from build123d import *

# Parameters (mm, degrees)
PAD_DEPTH    = 2
SKETCH001_R  = 4.2
POCKET_DEPTH = 1.1


with BuildPart() as part:
    # Sketch → Pad (new body)
    with BuildSketch(Plane.XY):
        with BuildLine():
            ThreePointArc((-47.293619, 36.923077), (0, -60), (47.293619, 36.923077))
            ThreePointArc((47.293619, 123.076923), (32.469508, 80), (47.293619, 36.923077))
            ThreePointArc((47.293619, 123.076923), (0, 220), (-47.293619, 123.076923))
            ThreePointArc((-47.293619, 36.923077), (-32.469508, 80), (-47.293619, 123.076923))
        make_face()
    extrude(amount=PAD_DEPTH)

    # Sketch001 (on Face6 of Pad) → Pocket (cut)
    with BuildSketch(Plane.XY.offset(2)):
        with Locations((0, -54.5)):
            Circle(SKETCH001_R)
        with Locations((0, 214.5)):
            Circle(SKETCH001_R)
        with Locations((0, 80)):
            Circle(SKETCH001_R)
    extrude(amount=-POCKET_DEPTH, mode=Mode.SUBTRACT)


solid = part.part
The listing builds one solid part. Answer for the finished solid, in the listing's coordinates (mm). A direction names the side the tool comes from. Round coordinates to 2 decimals unless told otherwise and drop trailing zeros. Write each loop counter-clockwise with the first axis right and the second up, starting at its lowest first coordinate (ties: lowest second). Pieces come first, ordered by that corner, then holes. Notation, with made-up numbers: (-35, 20.5) - (11, 20.5) arc R26 cw to (11, 48.5) - close; hole circle Ø4 at (61, 63). An arc over 180 degrees is marked (long way). Use a Markdown table: item, result. Add a question column.
1. The part is cut by section A-A (x = -52). Write down the section's boundary in (y, z), and give its area (3 significant figures).
2. The part is cut by section D-D (z = 0.4). Write down the section's boundary in (x, y).
3. The part is cut by section C-C (x = 0). Write down the section's boundary in (y, z), and give its area (3 significant figures).
4. Flat-ended cylindrical pins translate along their axes: P1, Ø4, axis at x = 1.5, y = 215.5, coming from the +Z side; P2, Ø4, axis at x = 18, y = -12, coming from the -Z side; P3, Ø1, axis at x = -47, z = 1.5, coming from the +Y side. Find the tip coordinate at first contact, or state that the pin passes through.
5. A tool of negligible diameter and unlimited length cuts with its end or side. For faces 3 (the face through (-1, 82, 0)), 4 (the face through (0, 215, 0.9)), from which of +Z, -Z, +X, -X, +Y, -Y can it reach the whole face along a straight path? Write none if from no direction.
6. The part is cut by section B-B (y = -54.5). Write down the section's boundary in (x, z).
7. For a pull along Y with two mould halves and no side action, classify faces 1 (the face through (12, 82, 2)), 2 (the face through (-0.91, 75.9, 1.46)) as +Y half, -Y half, draft (parallel to the pull), parting line (faces both ways), or undercut.
8. Consider line 1 (Y direction, x = 0, z = 1.4); line 2 (Y direction, x = 54, z = 1.05); line 3 (X direction, y = 170.5, z = 0.7). Determine where each line is inside the solid, lowest interval first.
Reported:
| question | item | result |
|---|---|---|
| 1 | outline | (-29.93, 0) - (29.93, 0) - (29.93, 2) - (-29.93, 2) - close; (130.07, 0) - (189.93, 0) - (189.93, 2) - (130.07, 2) - close |
| 1 | area | 239 mm^2 |
| 2 | outline | (-47.29, 36.92) arc R60 ccw (long way) to (47.29, 36.92) arc R70 cw to (47.29, 123.08) arc R60 ccw (long way) to (-47.29, 123.08) arc R70 cw to start |
| 3 | outline | (-60, 0) - (220, 0) - (220, 2) - (218.7, 2) - (218.7, 0.9) - (210.3, 0.9) - (210.3, 2) - (84.2, 2) - (84.2, 0.9) - (75.8, 0.9) - (75.8, 2) - (-50.3, 2) - (-50.3, 0.9) - (-58.7, 0.9) - (-58.7, 2) - (-60, 2) - close |
| 3 | area | 532 mm^2 |
| 4 | P1 | z = 0.9 |
| 4 | P2 | z = 0 |
| 4 | P3 | y = 197.92 |
| 5 | face 3 | -Z, +X, -X, +Y, -Y |
| 5 | face 4 | +Z |
| 6 | outline | (-25.09, 0) - (25.09, 0) - (25.09, 2) - (4.2, 2) - (4.2, 0.9) - (-4.2, 0.9) - (-4.2, 2) - (-25.09, 2) - close |
| 7 | face 1 | draft |
| 7 | face 2 | undercut |
| 8 | line 1 | -60 to -58.7, -50.3 to 75.8, 84.2 to 210.3, 218.7 to 220 |
| 8 | line 2 | -26.15 to 26.15, 133.85 to 186.15 |
| 8 | line 3 | -59.07 to 59.07 |
